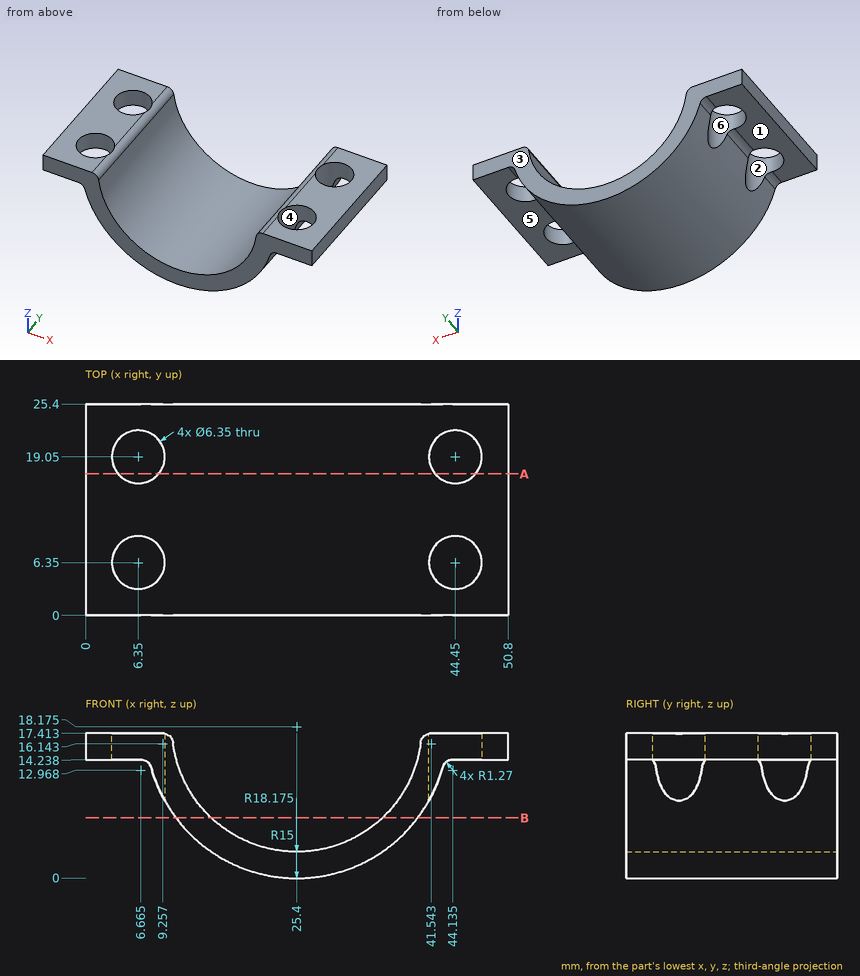
Can you work these out from the drawing? Everything is in mm from the part's minimum corner. A direction names the side the tool comes from. Give positions to 0.01 mm unless a question says otherwise; leave off trailing zeros. Order: outer loops, then holes, each group sorted by start corner. A loop starts at its lowest first (then second) coordinate and runs counter-clockwise, first axis right, second up. Notation, with made-up numbers: M -31,70 L 23,70 A12 ccw 23,86 Z; hole C -21.75,-21 d4. An arc over 180 degrees is marked long. Use a Markdown table: item, result. Add a question column.
1. Suppose I cut it at A-A (y = 17). Give the number of separate pieces and of enclosed holes in the cut face, and give its area (3 significant figures).
2. For pin 1 Ø4 at (y, z) = (22.5, 6.5) entering from +X (1 decimal); pin 2 Ø2 at (x, y) = (22, 10) entering from -Z; pin 3 Ø1 at (x, y) = (26.5, 21) entering from +Z, each with a flat end and sliding along its axis, tell me the tip position at first contact or that it passes through.
3. On a 3-axis mill with a long thin cutter (end or side, diameter ignored), from which of +Z, -Z, +X, -X, +Y, -Y can I reach the whole of each face in a straight line? I mean the marked faces 1 and 2. Say none if no direction works.
4. If we mould it in two halves opening along Y, with no side actions, what happens to the marked faces 3, 4, 5 and 6? For each: +Y half, -Y half, draft (parallel to the pull), parting line (faces both ways), or undercut.
5. Suppose I cut it at B-B (z = 7.25). List the corners of the cut face in (x, y) for me (1 decimal), and give its area (3 significant figures).
6. I need wall thicknesses on probe 1 along Y at (x, z) = (6.35, 14.5) (1 decimal); probe 2 along X at (y, z) = (18, 9.75) (1 decimal); probe 3 along Z at (x, y) = (2.5, 1.25). Which ranges of each line are inside material? Lowest first, please. Write a range as from..to.
Results list:
| question | item | result |
|---|---|---|
| 1 | separate pieces | 3 |
| 1 | enclosed holes | 0 |
| 1 | area | 172 mm² |
| 2 | pin 1 | stops at x = 40.8 |
| 2 | pin 2 | stops at z = 0.16 |
| 2 | pin 3 | stops at z = 3.26 |
| 3 | face 1 | -Z, -X, +Y, -Y |
| 3 | face 2 | +Z, -Z |
| 4 | face 3 | +Y half |
| 4 | face 4 | undercut |
| 4 | face 5 | draft |
| 4 | face 6 | undercut |
| 5 | outline | M 10.9,0 L 15.1,0 L 15.1,25.4 L 10.9,25.4 Z; M 35.7,0 L 39.9,0 L 39.9,25.4 L 35.7,25.4 Z |
| 5 | area | 216 mm² |
| 6 | probe 1 | y = 0..3.2, 9.5..15.9, 22.2..25.4 |
| 6 | probe 2 | x = 9.3..13, 37.8..41.5 |
| 6 | probe 3 | z = 14.24..17.41 |
